Work out the finished part from the listing and answer in its coordinate system (mm). Face numbers are marked on the shaded views. A direction names the side the tool comes from. Round coordinates to 2 decimals unless told otherwise and drop trailing zeros. Loops run counter-clockwise (first coordinate to the right, second up) from the corner with the lowest first, then second, coordinate; pieces in that order, holes last. Notation, with made-up numbers: (6, 8) - (44, 8) arc R23 cw to (44, 29) - close; hole circle Ø9 at (38, -4). An arc over 180 degrees is marked (long way). Return JSON: item names as keys, results as strings.
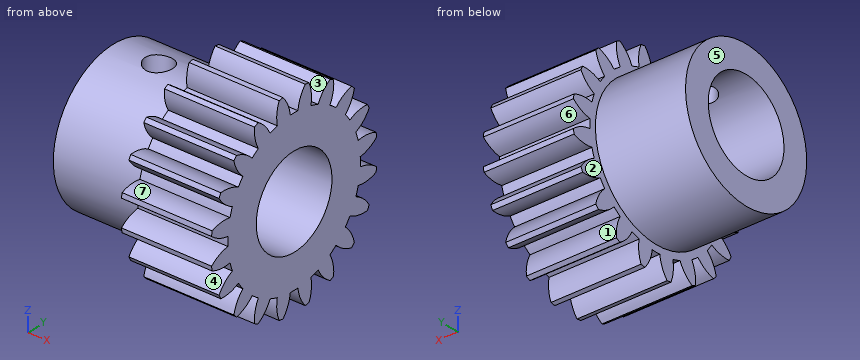
from build123d import *

# Parameters (mm, degrees)
BASPROSKE_W              = 10
BASPROSKE_H              = 11
TOOTHCUT_DEPTH           = 19.493242009
TEETHCUTS_COUNT          = 20
TEETHCUTS_ANGLE          = 342
HUBNEAONESKE_R           = 8
HUBNEARONE_DEPTH         = 10.0000508
BORSKE_R                 = 5
BORE_DEPTH               = 20.0000508
SKETCH_1_R               = 1.5
CUT_EXTRUDE_1_DEPTH      = 9
CUT_EXTRUDE_1_DEPTH_BACK = 1


with BuildPart() as part:
    # BasProSke → Base-Revolve (revolve)
    with BuildSketch(Plane(origin=(0, 0, 0), x_dir=(1, 0, 0), z_dir=(0, 1, 0)), mode=Mode.PRIVATE) as base_revolve_sk:
        with Locations((5, 5.5)):
            Rectangle(BASPROSKE_W, BASPROSKE_H)
    revolve(base_revolve_sk.sketch.rotate(Axis((-10, 0, 0), (1, 0, 0)), 180), axis=Axis((-10, 0, 0), (1, 0, 0)))

    # TooCutSke → ToothCut (cut, through all)
    with BuildSketch(Plane(origin=(0, 0, 0), x_dir=(0, 0, -1), z_dir=(1, 0, 0))):
        with BuildLine():
            ThreePointArc((0.499924007, 8.734705318), (0, 8.749), (-0.499924007, 8.734705318))
            ThreePointArc((-0.499924007, 8.734705318), (-0.824302243, 9.905497836), (-1.485192705, 10.924909509))
            ThreePointArc((-1.485192705, 10.924909509), (0, 11.0254), (1.485192705, 10.924909509))
            ThreePointArc((1.485192705, 10.924909509), (0.824302243, 9.905497836), (0.499924007, 8.734705318))
        make_face()
    toothcut = extrude(amount=TOOTHCUT_DEPTH, mode=Mode.SUBTRACT)

    # TeethCuts: ToothCut ×20 about axis
    teethcuts_axis = Axis((-10, 0, 0), (1, 0, 0))
    for i in range(1, TEETHCUTS_COUNT):
        add(toothcut.rotate(teethcuts_axis, i * TEETHCUTS_ANGLE / (TEETHCUTS_COUNT - 1)), mode=Mode.SUBTRACT)

    # HubNeaOneSke → HubNearOne (add)
    with BuildSketch(Plane.ZY):
        with Locations(Location((0, 0, 0), (0, 0, 180))):
            Circle(HUBNEAONESKE_R)
    extrude(amount=HUBNEARONE_DEPTH)

    # BorSke → Bore (cut, symmetric)
    with BuildSketch(Plane(origin=(0, 0, 0), x_dir=(0, 0, -1), z_dir=(1, 0, 0))):
        with Locations(Location((0, 0, 0), (0, 0, 180))):
            Circle(BORSKE_R)
    extrude(amount=BORE_DEPTH, both=True, mode=Mode.SUBTRACT)

    # 草图1 → 切除-拉伸1 (cut, two sides)
    with BuildSketch(Plane.XY) as cut_extrude_1_sk:
        with Locations(Location((-5.0000508, 0, 0), (0, 0, 180.000000001))):
            Circle(SKETCH_1_R)
    extrude(amount=CUT_EXTRUDE_1_DEPTH, mode=Mode.SUBTRACT)
    extrude(cut_extrude_1_sk.sketch, amount=-CUT_EXTRUDE_1_DEPTH_BACK, mode=Mode.SUBTRACT)


solid = part.part
1) Find the intervals of material crossed by L1, parallel to X at y = 0, z = 7.3; L2, parallel to Z at x = 2.25, y = 7.5; L3, parallel to Z at x = 6.5, y = 9, in increasing order.
Verdict:
{"L1": "x = -10 to -6.5, -3.5 to 10", "L2": "z = -7.94 to -6.44, -4.8 to 4.8, 6.44 to 7.94", "L3": "z = -5.23 to -3.7, -2.29 to -0.54, 0.54 to 2.29, 3.7 to 5.23"}
2) Determine the mould class of the marked faces 4, 5, 6 and 7 for opening direction Y: pulls with the +Y half, pulls with the -Y half, needs draft (parallel to the pull), parting line crosses it, or undercut.
Verdict:
{"face 4": "pulls with the -Y half", "face 5": "needs draft", "face 6": "pulls with the +Y half", "face 7": "undercut"}
3) Section A-A (z = 0) is taken. Give the vertices of the cut face in (x, y).
Verdict:
{"outline": "(-10, -8) - (0, -8) - (0, -8.75) - (10, -8.75) - (10, -5) - (-10, -5) - close; (-10, 5) - (10, 5) - (10, 8.75) - (0, 8.75) - (0, 8) - (-10, 8) - close"}
4) A tool of negligible diameter and unlimited length cuts with its end or side. For the marked faces 1, 2 and 3, from which of +Z, -Z, +X, -X, +Y, -Y can it reach the whole face along a straight path? Write none if from no direction.
Verdict:
{"face 1": "+X, -X", "face 2": "-X", "face 3": "+Z, +X, -X"}
5) Flat-ended cylindrical pins translate along their axes: pin 1 (6 mm diameter, centred on x = -5, y = -4.5, fed in from -Z); pin 2 (3.5 mm diameter, centred on x = -5, y = 0, fed in from +Z); pin 3 (8 mm diameter, centred on x = -1.5, z = -6, fed in from -Y); pin 4 (9 mm diameter, centred on y = 0, z = 0, fed in from -X). Find the tip coordinate at first contact, or state that the pin passes through.
Verdict:
{"pin 1": "stops at z = -7.86", "pin 2": "stops at z = 8", "pin 3": "stops at y = -9.92", "pin 4": "passes through"}
6) Section B-B (y = 0) is taken. Give the vertices of the cut face in (x, z).
Verdict:
{"outline": "(-10, -8) - (0, -8) - (0, -8.75) - (10, -8.75) - (10, -5) - (-10, -5) - close; (-10, 5) - (-6.5, 5) - (-6.5, 8) - (-10, 8) - close; (-3.5, 5) - (10, 5) - (10, 8.75) - (0, 8.75) - (0, 8) - (-3.5, 8) - close"}
7) Section C-C (x = -2.75) is taken. Give the vertices of the cut face in (y, z).
Verdict:
{"outline": "circle Ø16 at (0, 0); hole circle Ø10 at (0, 0)"}
